Build history of the part. All positions in model axes, mm. Face numbers are marked on the shaded views. Give positions to 0.01 mm unless a question says otherwise; leave off trailing zeros. Order: outer loops, then holes, each group sorted by start corner. A loop starts at its lowest first (then second) coordinate and runs counter-clockwise, first axis right, second up. Notation, with made-up numbers: (58, 31) - (99, 31) arc R18 cw to (99, 64) - close; hole circle Ø10 at (49, 31.25). An arc over 180 degrees is marked (long way). Write each question's results on one line, items separated by ' | '. Start each with the question number.
1) Cut at D-D on z = -25.5. List the corners of the cut face in (x, y).
2) Cut at C-C on x = 48. List the corners of the cut face in (y, z), plus the area to 3 significant figures.
3) Cut at A-A on y = 2. State how many separate pieces and enclosed holes the cut face has, plus the area to 3 significant figures.
4) Drill centre lines: line 1 along X through (y, z) = (1.85, -2); line 2 along X through (y, z) = (1.25, -23); line 3 along Z through (x, y) = (55, 3.8). Where is each one in solid material? Low to high. Write a range as from..to.
5) Cut at B-B on z = -16. List the corners of the cut face in (x, y).
6) Drop flat-ended pins along their axis: pin 1 Ø6 at (x, z) = (22, -11.5) entering from +Y; pin 2 Ø1.8 at (x, z) = (38.5, -22.5) entering from +Y. Give the stop position or say it passes through.
7) Two-plate mould, pull along X, no slides. Class the marked faces 1 and 2: +X half, -X half, draft (parallel to the pull), parting line (faces both ways), or undercut.
from build123d import *

# Parameters (mm, degrees)
SKETCH2_W           = 60.65
SKETCH2_H           = 36.2
BOSS_EXTRUDE1_DEPTH = 1.2
SKETCH3_W           = 60.65
SKETCH3_H           = 36.2
SKETCH3_W_2         = 58.25
SKETCH3_H_2         = 33.8
BOSS_EXTRUDE2_DEPTH = 3.3
SKETCH4_W           = 16
SKETCH4_H           = 6
SKETCH4_W_2         = 5.5
SKETCH4_H_2         = 10.5
SKETCH4_W_3         = 11
SKETCH4_H_3         = 4.5
SKETCH4_W_4         = 15
SKETCH4_W_5         = 5
SKETCH4_H_4         = 14
SKETCH4_W_6         = 8.2
SKETCH4_W_7         = 6
BOSS_EXTRUDE3_DEPTH = 1.8


with BuildPart() as part:
    # Sketch2 → Boss-Extrude1 (new body)
    with BuildSketch(Plane(origin=(0, 0, 0), x_dir=(1, 0, 0), z_dir=(0, 1, 0))):
        with Locations((29.125, 16.9)):
            Rectangle(SKETCH2_W, SKETCH2_H)
    extrude(amount=BOSS_EXTRUDE1_DEPTH)

    # Sketch3 → Boss-Extrude2 (add)
    with BuildSketch(Plane(origin=(0, 1.2, 0), x_dir=(1, 0, 0), z_dir=(0, 1, 0))):
        with Locations((29.125, 16.9)):
            Rectangle(SKETCH3_W, SKETCH3_H)
        with Locations((29.125, 16.9)):
            Rectangle(SKETCH3_W_2, SKETCH3_H_2, mode=Mode.SUBTRACT)
    extrude(amount=BOSS_EXTRUDE2_DEPTH)

    # Sketch4 → Boss-Extrude3 (add)
    with BuildSketch(Plane(origin=(0, 1.2, 0), x_dir=(1, 0, 0), z_dir=(0, 1, 0))):
        with Locations((8, 30.8)):
            Rectangle(SKETCH4_W, SKETCH4_H)
        with Locations((2.75, 10.05)):
            Rectangle(SKETCH4_W_2, SKETCH4_H_2)
        with Locations((39.75, 2.25)):
            Rectangle(SKETCH4_W_3, SKETCH4_H_3)
        with Locations((13.5, 2.25)):
            Rectangle(SKETCH4_W_4, SKETCH4_H_3)
        with Locations((55.75, 12.5)):
            Rectangle(SKETCH4_W_5, SKETCH4_H_4)
        with Locations((26.1, 30.8)):
            Rectangle(SKETCH4_W_6, SKETCH4_H)
        with Locations((37.29, 21.13)):
            Rectangle(SKETCH4_W_7, SKETCH4_H)
    extrude(amount=BOSS_EXTRUDE3_DEPTH)


solid = part.part
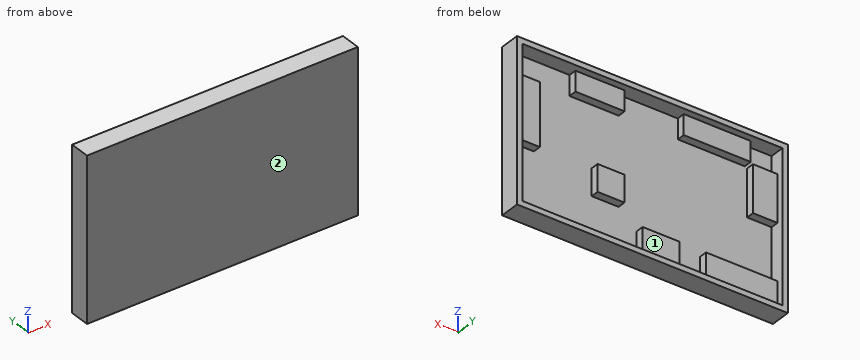
Results:
1) outline: (-1.2, 0) - (59.45, 0) - (59.45, 4.5) - (58.25, 4.5) - (58.25, 1.2) - (0, 1.2) - (0, 4.5) - (-1.2, 4.5) - close
2) outline: (0, -35) - (4.5, -35) - (4.5, -33.8) - (1.2, -33.8) - (1.2, 0) - (4.5, 0) - (4.5, 1.2) - (0, 1.2) - close | area: 51.4 mm^2
3) separate pieces: 2 | enclosed holes: 1 | area: 653 mm^2
4) line 1: -1.2..0, 6..21, 34.25..45.25, 58.25..59.45 | line 2: -1.2..0, 34.29..40.29, 58.25..59.45 | line 3: -35..-33.8, 0..1.2
5) outline: (-1.2, 0) - (59.45, 0) - (59.45, 4.5) - (58.25, 4.5) - (58.25, 3) - (53.25, 3) - (53.25, 1.2) - (0, 1.2) - (0, 4.5) - (-1.2, 4.5) - close
6) pin 1: y = 1.2 | pin 2: y = 3
7) face 1: undercut | face 2: draft
